Read the model definition and answer for the solid it produces. Units are mm, in the model's axes. A direction names the side the tool comes from. Round coordinates to 2 decimals unless told otherwise and drop trailing zeros. Order: outer loops, then holes, each group sorted by start corner. A loop starts at its lowest first (then second) coordinate and runs counter-clockwise, first axis right, second up. Notation, with made-up numbers: (53, 24) - (100, 24) arc R26 cw to (100, 59) - close; hole circle Ø5 at (45, 4.25). An arc over 180 degrees is marked (long way). One line per question, with ' | ' between items. Start each with the question number.
1) Straight lines are drawn through the part: line 1 (X direction, y = 12.25, z = 0) (3 decimals); line 2 (X direction, y = 10, z = 0) (3 decimals); line 3 (X direction, y = 3.75, z = 0) (3 decimals). For each, find the intervals that lie inside material, in ascending order. Write a range as from..to.
2) The part is cut by section C-C, the plane y = 7. Give the vertices of the cut face in (x, z) (3 decimals).
3) The part is cut by section D-D, the plane x = -1. Give the vertices of the cut face in (y, z).
4) The part is cut by section B-B, the plane x = 87.5. Give the vertices of the cut face in (y, z), plus the area to 3 significant figures.
5) The part is cut by section A-A, the plane y = 1.5. Give the vertices of the cut face in (x, z) (3 decimals), plus the area to 3 significant figures.
6) For faces 5 (the flat face through (5.46, 11.58, -0.74)), 6 (the flat face through (64, 2, -6.35)), 7 (the cylindrical face through (-0.74, -7.89, 2.36)), determine the directions among +Z, -Z, +X, -X, +Y, -Y from which every point of the face is accessible in a straight line to the end or side of a thin tool.
7) The mould has two halves that part along X. Classify faces 1 (the cylindrical face through (-8.35, 2.46, 0.18)), 2 (the flat face through (56.325, 2, 0)), 3 (the flat face through (86, 15, 0)), 4 (the cylindrical face through (4.34, 11.58, -7.47)): pulls with the +X half, pulls with the -X half, needs draft (parallel to the pull), parting line crosses it, or undercut.
8) Flat-ended cylindrical pins translate along their axes: pin 1 (6 mm diameter, centred on x = 45, z = 2.5, fed in from -Y); pin 2 (8.5 mm diameter, centred on x = 50, z = -2, fed in from +Y); pin 3 (1.5 mm diameter, centred on y = 2.5, z = -2.5, fed in from +X); pin 4 (6.5 mm diameter, centred on x = 90, z = 0, fed in from -Y). Find the tip coordinate at first contact, or state that the pin passes through.
from build123d import *

# Parameters (mm, degrees)
CORPS_DEPTH             = 5
ESQUISSE1_R             = 2.475
PULLEY_HOLD_DEPTH       = 16
ESQUISSE2_R             = 4
KNOB_HOLD_DEPTH         = 8.1
KNOB_START              = 5.1
KNOB_DEPTH              = 3
ESQUISSE3_R             = 3.675
ESQUISSE3_W             = 15
ESQUISSE3_H             = 12.7
ENL_V_MAT_EXTRU_1_DEPTH = 100.992224698
ESQUISSE5_R             = 4.675
ESQUISSE5_R_2           = 3.675
BOSS_EXTRU_1_DEPTH      = 10


with BuildPart() as part:
    # Sketch1 → corps (new body)
    with BuildSketch(Plane(origin=(0, 0, 0), x_dir=(1, 0, 0), z_dir=(0, 1, 0))):
        with BuildLine():
            Line((0, 8.35), (90, 8.35))
            ThreePointArc((90, 8.35), (98.35, 0), (90, -8.35))
            Line((90, -8.35), (0, -8.35))
            ThreePointArc((0, -8.35), (-8.35, 0), (0, 8.35))
        make_face()
    extrude(amount=CORPS_DEPTH)

    # Esquisse1 → pulley hold (add)
    with BuildSketch(Plane.XZ):
        with Locations(Location((0, 0, 0), (0, 0, 90))):
            Circle(ESQUISSE1_R)
    extrude(amount=PULLEY_HOLD_DEPTH)

    # Esquisse2 → knob hold (add)
    with BuildSketch(Plane(origin=(0, 5, 0), x_dir=(1, 0, 0), z_dir=(0, 1, 0))):
        with Locations(Location((0, 0, 0), (0, 0, 270))):
            Circle(ESQUISSE2_R)
    extrude(amount=KNOB_HOLD_DEPTH)

    # Esquisse4 → knob (add)
    with BuildSketch(Plane(origin=(0, 5, 0), x_dir=(1, 0, 0), z_dir=(0, 1, 0)).offset(KNOB_START)):
        with BuildLine():
            Line((3.999579917, 0.057969697), (6.953398299, 1.435357829))
            ThreePointArc((6.953398299, 1.435357829), (7.074856515, 0.596996899), (7.095602071, -0.249862457))
            ThreePointArc((7.095602071, -0.249862457), (8.44546622, -1.698263913), (9.893867677, -0.348399764))
            ThreePointArc((9.893867677, -0.348399764), (9.026569148, 4.065839324), (6.295408565, 7.640538659))
            ThreePointArc((6.295408565, 7.640538659), (4.324668554, 7.450318241), (4.514888971, 5.47957823))
            ThreePointArc((4.514888971, 5.47957823), (5.06564099, 4.974864959), (5.560313894, 4.415077508))
            Line((5.560313894, 4.415077508), (2.603837765, 3.036450048))
            ThreePointArc((2.603837765, 3.036450048), (3.622032243, 1.697316243), (3.999579917, 0.057969697))
        make_face()
    extrude(amount=KNOB_DEPTH)

    # Esquisse3 → Enlèv. mat.-Extru.1 (cut, through all)
    with BuildSketch(Plane.XZ):
        with Locations(Location((90, 0, 0), (0, 0, 270))):
            Circle(ESQUISSE3_R)
        with Locations((63.825, 0)):
            Rectangle(ESQUISSE3_W, ESQUISSE3_H)
    extrude(amount=-ENL_V_MAT_EXTRU_1_DEPTH, mode=Mode.SUBTRACT)

    # Esquisse5 → Boss.-Extru.1 (add)
    with BuildSketch(Plane(origin=(0, 5, 0), x_dir=(1, 0, 0), z_dir=(0, 1, 0))):
        with Locations(Location((90, 0, 0), (0, 0, 270))):
            Circle(ESQUISSE5_R)
        with Locations(Location((90, 0, 0), (0, 0, 90))):
            Circle(ESQUISSE5_R_2, mode=Mode.SUBTRACT)
    extrude(amount=BOSS_EXTRU_1_DEPTH)


solid = part.part
Values:
1) line 1: x = -4..4, 7.1..9.9, 85.325..86.325, 93.675..94.675 | line 2: x = -4..4, 85.325..86.325, 93.675..94.675 | line 3: x = -8.35..56.325, 71.325..86.325, 93.675..98.35
2) outline: circle Ø8 at (0, 0); circle Ø9.35 at (90, 0); hole circle Ø7.35 at (90, 0)
3) outline: (-16, -2.26) - (0, -2.26) - (0, -8.29) - (5, -8.29) - (5, -3.87) - (13.1, -3.87) - (13.1, 3.87) - (5, 3.87) - (5, 8.29) - (0, 8.29) - (0, 2.26) - (-16, 2.26) - close
4) outline: (0, -8.35) - (5, -8.35) - (5, -3.95) - (15, -3.95) - (15, -2.69) - (0, -2.69) - close; (0, 2.69) - (15, 2.69) - (15, 3.95) - (5, 3.95) - (5, 8.35) - (0, 8.35) - close | area: 81.7 mm^2
5) outline: (0, -8.35) - (90, -8.35) arc R8.35 ccw to (90, 8.35) - (0, 8.35) arc R8.35 ccw to start; hole (56.325, -6.35) - (71.325, -6.35) - (71.325, 6.35) - (56.325, 6.35) - close; hole circle Ø7.35 at (90, 0) | area: 1,490 mm^2
6) face 5: +Z, +Y | face 6: +Y, -Y | face 7: -Y
7) face 1: pulls with the -X half | face 2: undercut | face 3: needs draft | face 4: parting line crosses it
8) pin 1: stops at y = 0 | pin 2: stops at y = 5 | pin 3: stops at x = 98.16 | pin 4: passes through
